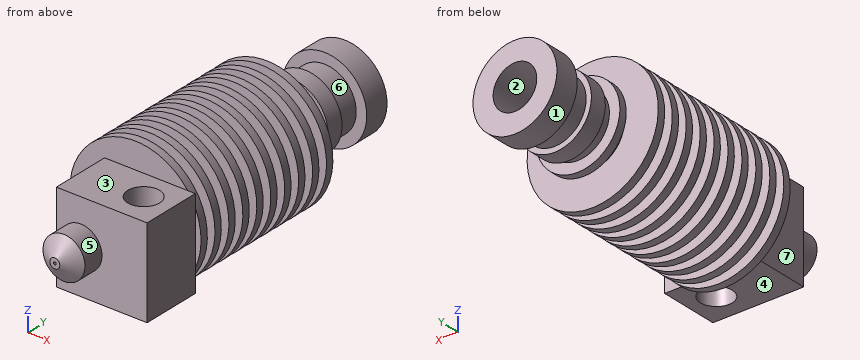
```python
from build123d import *

# Parameters (mm, degrees)
SKETCH2_R           = 4.159262234
CUT_EXTRUDE1_DEPTH  = 10
SKETCH3_W           = 17.293974885
SKETCH3_H           = 11.410212081
BOSS_EXTRUDE1_DEPTH = 8.5
SKETCH4_R           = 3.04865438
CUT_EXTRUDE2_DEPTH  = 17


with BuildPart() as part:
    # Sketch1 → Revolve1 (revolve)
    with BuildSketch(Plane.XY, mode=Mode.PRIVATE) as revolve1_sk:
        Polygon((-2, -15.925549295), (-2, -28.816393339), (-4, -28.816393339), (-4, -32.836590434), (-0.942955999, -34.998102919), (-0.25, -34.998102919), (-0.25, -33.674450705), (0, -33.674450705), (0, 33.674450705), (-8, 33.674450705), (-8, 28.874450705), (-6, 28.874450705), (-6, 24.274450705), (-7, 24.274450705), (-7, 20.974450705), (-6, 20.974450705), (-6, 18.774450705), (-8, 18.774450705), (-8, 17.274450705), (-6, 17.274450705), (-6, 15.274450705), (-12.5, 15.274450705), (-12.5, 13.774450705), (-7.5, 13.774450705), (-7.5, 11.974450705), (-12.5, 11.974450705), (-12.5, 10.474450705), (-7.5, 10.474450705), (-7.5, 8.674450705), (-12.5, 8.674450705), (-12.5, 7.174450705), (-7.5, 7.174450705), (-7.5, 5.374450705), (-12.5, 5.374450705), (-12.5, 3.874450705), (-7.5, 3.874450705), (-7.5, 2.074450705), (-12.5, 2.074450705), (-12.5, 0.574450705), (-7.5, 0.574450705), (-7.5, -1.225549295), (-12.5, -1.225549295), (-12.5, -2.725549295), (-7.5, -2.725549295), (-7.5, -4.525549295), (-12.5, -4.525549295), (-12.5, -6.025549295), (-7.5, -6.025549295), (-7.5, -7.825549295), (-12.5, -7.825549295), (-12.5, -9.325549295), (-7.5, -9.325549295), (-7.5, -11.125549295), (-12.5, -11.125549295), (-12.5, -12.625549295), (-7.5, -12.625549295), (-7.5, -14.425549295), (-12.5, -14.425549295), (-12.5, -15.925549295), align=None)
    revolve(revolve1_sk.sketch.rotate(Axis((0, -1005.655436074, 0), (0, 1, 0)), 270), axis=Axis((0, -1005.655436074, 0), (0, 1, 0)))

    # Sketch2 → Cut-Extrude1 (cut)
    with BuildSketch(Plane(origin=(0, 33.674450705, 0), x_dir=(1, 0, 0), z_dir=(0, 1, 0))):
        with Locations(Location((0, 0, 0), (0, 0, 270))):
            Circle(SKETCH2_R)
    extrude(amount=-CUT_EXTRUDE1_DEPTH, mode=Mode.SUBTRACT)

    # Sketch3 → Boss-Extrude1 (add, symmetric)
    with BuildSketch(Plane.XY):
        with Locations((3.80447813, -22.923519592)):
            Rectangle(SKETCH3_W, SKETCH3_H)
    extrude(amount=BOSS_EXTRUDE1_DEPTH, both=True)

    # Sketch4 → Cut-Extrude2 (cut)
    with BuildSketch(Plane.XY.offset(8.5)):
        with Locations((7.066076907, -22.750382856)):
            Circle(SKETCH4_R)
    extrude(amount=-CUT_EXTRUDE2_DEPTH, mode=Mode.SUBTRACT)


solid = part.part
```
For this review, take the finished solid that the model builds, in its own axes (mm). Face numbers are marked on the shaded views. A direction names the side the tool comes from. Coordinates: 2 decimals unless noted, no trailing zeros. Write each loop counter-clockwise with the first axis right and the second up, starting at its lowest first coordinate (ties: lowest second). Pieces come first, ordered by that corner, then holes.
(1) Tool access review of the marked faces 4, 5, 6 and 7: name each direction out of +Z, -Z, +X, -X, +Y, -Y from which nothing blocks a thin tool from reaching the whole face with its end or side.
(2) Wall thickness on probe 1 along Y at (x, z) = (-2.25, 5.75); probe 2 along X at (y, z) = (27.25, 0); probe 3 along Y at (x, z) = (-2, -4.5): over which ranges is each line inside the solid? List them lowest first.
(3) Add section B-B on x = -10.5. Count the separate pieces of the cut face and the enclosed holes in it, then the cut area to 3 significant figures.
(4) The part is to be moulded in two halves that separate along X. For the marked faces 1, 2 and 3, say which applies: +X half, -X half, draft (parallel to the pull), parting line (faces both ways), or undercut.
(5) For pin 1 Ø6 at (y, z) = (-13, 6.5) entering from -X; pin 2 Ø12 at (x, z) = (8.5, -10) entering from +Y; pin 3 Ø4 at (x, z) = (-0.5, 1) entering from +Y; pin 4 Ø5.5 at (y, z) = (-25.5, -0.5) entering from -X, all flat-tipped, find the tip position at first contact; note any pin that passes through.
(6) Add section A-A on y = -7. Give the boundary of the cut face in (x, z).
Answer sheet:
1. face 4: -Z, +X, -X, -Y
1. face 5: -Y
1. face 6: none
1. face 7: +Z, -Z, -X, -Y
2. probe 1: y = -28.63 to -17.22, -15.93 to 15.27, 17.27 to 18.77, 20.97 to 24.27, 28.87 to 33.67
2. probe 2: x = -6 to -4.16, 4.16 to 6
2. probe 3: y = -28.63 to -17.22, -15.93 to 33.67
3. separate pieces: 10
3. enclosed holes: 0
3. area: 203 mm2
4. face 1: parting line
4. face 2: undercut
4. face 3: draft
5. pin 1: stops at x = -11.99
5. pin 2: stops at y = 33.67
5. pin 3: stops at y = 23.67
5. pin 4: stops at x = -4.84
6. outline: circle Ø15 at (0, 0)
